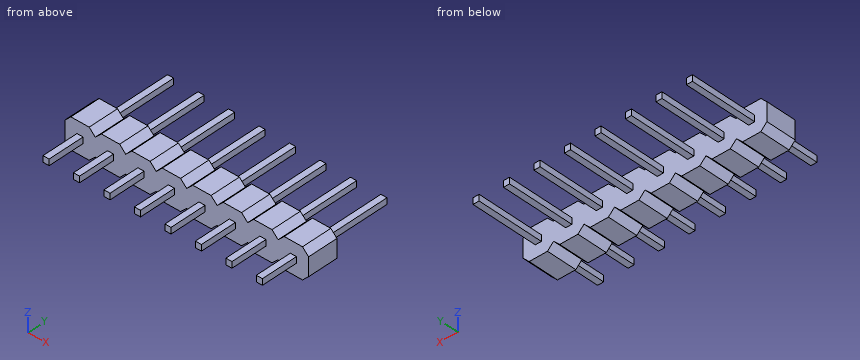
```python
from build123d import *

# Parameters (mm, degrees)
BOSS_EXTRUDE1_DEPTH = 2.5
SKETCH2_W           = 0.5
SKETCH2_H           = 0.5
BOSS_EXTRUDE2_DEPTH = 5.5
SKETCH2_2_W         = 0.5
SKETCH2_2_H         = 0.5
BOSS_EXTRUDE3_DEPTH = 5.5


with BuildPart() as part:
    # Sketch1 → Boss-Extrude1 (new body)
    with BuildSketch(Plane(origin=(0, 0, 0), x_dir=(1, 0, 0), z_dir=(0, 1, 0))):
        Polygon((-1.25, 0.75), (-0.75, 1.25), (0.75, 1.25), (1.25, 0.75), (1.75, 1.25), (3.25, 1.25), (3.75, 0.75), (4.25, 1.25), (5.75, 1.25), (6.25, 0.75), (6.75, 1.25), (8.25, 1.25), (8.75, 0.75), (9.25, 1.25), (10.75, 1.25), (11.25, 0.75), (11.75, 1.25), (13.25, 1.25), (13.75, 0.75), (14.25, 1.25), (15.75, 1.25), (16.25, 0.75), (16.75, 1.25), (18.25, 1.25), (18.75, 0.75), (18.75, -0.75), (18.25, -1.25), (16.75, -1.25), (16.25, -0.75), (15.75, -1.25), (14.25, -1.25), (13.75, -0.75), (13.25, -1.25), (11.75, -1.25), (11.25, -0.75), (10.75, -1.25), (9.25, -1.25), (8.75, -0.75), (8.25, -1.25), (6.75, -1.25), (6.25, -0.75), (5.75, -1.25), (4.25, -1.25), (3.75, -0.75), (3.25, -1.25), (1.75, -1.25), (1.25, -0.75), (0.75, -1.25), (-0.75, -1.25), (-1.25, -0.75), align=None)
    extrude(amount=BOSS_EXTRUDE1_DEPTH)

    # Sketch2 → Boss-Extrude2 (add)
    with BuildSketch(Plane(origin=(0, 2.5, 0), x_dir=(1, 0, 0), z_dir=(0, 1, 0))):
        with Locations((2.5, 0)):
            Rectangle(SKETCH2_W, SKETCH2_H)
        Rectangle(SKETCH2_W, SKETCH2_H)
        with Locations((5, 0)):
            Rectangle(SKETCH2_W, SKETCH2_H)
        with Locations((7.5, 0)):
            Rectangle(SKETCH2_W, SKETCH2_H)
        with Locations((10, 0)):
            Rectangle(SKETCH2_W, SKETCH2_H)
        with Locations((12.5, 0)):
            Rectangle(SKETCH2_W, SKETCH2_H)
        with Locations((15, 0)):
            Rectangle(SKETCH2_W, SKETCH2_H)
        with Locations((17.5, 0)):
            Rectangle(SKETCH2_W, SKETCH2_H)
    extrude(amount=BOSS_EXTRUDE2_DEPTH)

    # Sketch2<2> → Boss-Extrude3 (add)
    with BuildSketch(Plane(origin=(0, 2.5, 0), x_dir=(1, 0, 0), z_dir=(0, 1, 0))):
        with Locations((2.5, 0)):
            Rectangle(SKETCH2_2_W, SKETCH2_2_H)
        Rectangle(SKETCH2_2_W, SKETCH2_2_H)
        with Locations((5, 0)):
            Rectangle(SKETCH2_2_W, SKETCH2_2_H)
        with Locations((7.5, 0)):
            Rectangle(SKETCH2_2_W, SKETCH2_2_H)
        with Locations((10, 0)):
            Rectangle(SKETCH2_2_W, SKETCH2_2_H)
        with Locations((12.5, 0)):
            Rectangle(SKETCH2_2_W, SKETCH2_2_H)
        with Locations((15, 0)):
            Rectangle(SKETCH2_2_W, SKETCH2_2_H)
        with Locations((17.5, 0)):
            Rectangle(SKETCH2_2_W, SKETCH2_2_H)
    extrude(amount=-BOSS_EXTRUDE3_DEPTH)


solid = part.part
```
Model file for the job. Use its own axes, mm. Coordinates: 2 decimals unless noted, no trailing zeros. Order: outer loops, then holes, each group sorted by start corner. A loop starts at its lowest first (then second) coordinate and runs counter-clockwise, first axis right, second up. Notation, with made-up numbers: (69.25, 56) - (109.25, 56) arc R31 cw to (109.25, 94) - close; hole circle Ø1 at (45.5, 13). An arc over 180 degrees is marked (long way). Return JSON: item names as keys, results as strings. Group by question number.
1) Flat gauge pins, fed straight in: P1, Ø3, axis at x = 4, y = 6.5, coming from the -Z side; P2, Ø0.6, axis at y = 4.5, z = 0, coming from the +X side; P3, Ø0.6, axis at x = 2.5, y = 4, coming from the +Z side. Where does each tip first touch, or does it go through?
2) Saw through at A-A, the plane z = 1. Count the separate pieces of the cut face and the enclosed holes in it, plus the area to 3 significant figures.
3) Saw through at D-D, the plane x = 17. Write the cut outline in (y, z).
4) Probe line 1 (Y direction, x = 2, z = 0.8). List the from-to ranges inside material, lowest first. Write a range as from..to.
5) Saw through at C-C, the plane x = 14. Write the cut outline in (y, z), plus the area to 3 significant figures.
Values found:
{
 "1": {"P1": "stops at z = -0.25", "P2": "stops at x = 17.75", "P3": "stops at z = 0.25"},
 "2": {"separate pieces": "8", "enclosed holes": "0", "area": "40.0 mm²"},
 "3": {"outline": "(0, -1.25) - (2.5, -1.25) - (2.5, 1.25) - (0, 1.25) - close"},
 "4": {"line 1": "y = 0..2.5"},
 "5": {"outline": "(0, -1) - (2.5, -1) - (2.5, 1) - (0, 1) - close", "area": "5.00 mm²"}
}
